Build history of the part. All positions in model axes, mm. A direction names the side the tool comes from. Give positions to 0.01 mm unless a question says otherwise; leave off trailing zeros. Use a Markdown table: item, result. Add a question column.
```python
from build123d import *

# Parameters (mm, degrees)
SKETCH1_R           = 1.5
SKETCH1_R_2         = 1.25
SKETCH1_R_3         = 2.05
BOSS_EXTRUDE1_DEPTH = 2
FILLET7_R           = 8
BOSS_EXTRUDE2_DEPTH = 2
FILLET8_R           = 10
SKETCH4_R           = 1.55
CUT_EXTRUDE1_DEPTH  = 2
SKETCH5_R           = 1.55
CUT_EXTRUDE2_DEPTH  = 2
CUT_EXTRUDE3_DEPTH  = 10
SKETCH7_R           = 1.5
CUT_EXTRUDE4_DEPTH  = 10


with BuildPart() as part:
    # Sketch1 → Boss-Extrude1 (new body)
    with BuildSketch(Plane.XY):
        with BuildLine():
            Line((-86.974134086, 60.104076401), (-60.104076401, 86.974134086))
            Line((-60.104076401, 86.974134086), (60.104076401, 86.974134086))
            Line((60.104076401, 86.974134086), (86.974134086, 60.104076401))
            ThreePointArc((86.974134086, 60.104076401), (73.41582025, 0), (86.974134086, -60.104076401))
            Line((86.974134086, -60.104076401), (60.104076401, -86.974134086))
            Line((60.104076401, -86.974134086), (-60.104076401, -86.974134086))
            Line((-60.104076401, -86.974134086), (-86.974134086, -60.104076401))
            ThreePointArc((-86.974134086, -60.104076401), (-73.41582025, 0), (-86.974134086, 60.104076401))
        make_face()
        with Locations((-15, 57.5)):
            Circle(SKETCH1_R, mode=Mode.SUBTRACT)
        with Locations((-15, 27.5)):
            Circle(SKETCH1_R, mode=Mode.SUBTRACT)
        with Locations((15, 27.5)):
            Circle(SKETCH1_R, mode=Mode.SUBTRACT)
        with Locations((15, 57.5)):
            Circle(SKETCH1_R, mode=Mode.SUBTRACT)
        with Locations((-24, -13.5)):
            Circle(SKETCH1_R_2, mode=Mode.SUBTRACT)
        with Locations((24, -13.5)):
            Circle(SKETCH1_R_2, mode=Mode.SUBTRACT)
        with Locations((24, -46.5)):
            Circle(SKETCH1_R_2, mode=Mode.SUBTRACT)
        with Locations((-24, -46.5)):
            Circle(SKETCH1_R_2, mode=Mode.SUBTRACT)
        with Locations((-76.190755673, 58.159532753)):
            Circle(SKETCH1_R_3, mode=Mode.SUBTRACT)
        with Locations((-58.159532753, 76.190755673)):
            Circle(SKETCH1_R_3, mode=Mode.SUBTRACT)
        with Locations((76.190755673, -58.159532753)):
            Circle(SKETCH1_R_3, mode=Mode.SUBTRACT)
        with Locations((58.159532753, -76.190755673)):
            Circle(SKETCH1_R_3, mode=Mode.SUBTRACT)
        with Locations((-58.159532753, -76.190755673)):
            Circle(SKETCH1_R_3, mode=Mode.SUBTRACT)
        with Locations((-76.190755673, -58.159532753)):
            Circle(SKETCH1_R_3, mode=Mode.SUBTRACT)
        with Locations((58.159532753, 76.190755673)):
            Circle(SKETCH1_R_3, mode=Mode.SUBTRACT)
        with Locations((76.190755673, 58.159532753)):
            Circle(SKETCH1_R_3, mode=Mode.SUBTRACT)
    extrude(amount=BOSS_EXTRUDE1_DEPTH)

    # Fillet7
    fillet7_edges = [part.edges().sort_by_distance(p)[0] for p in [
        (86.974134086, -60.104076401, 1),
        (60.104076401, -86.974134086, 1),
        (-60.104076401, -86.974134086, 1),
        (-86.974134086, -60.104076401, 1),
        (-86.974134086, 60.104076401, 1),
        (-60.104076401, 86.974134086, 1),
        (60.104076401, 86.974134086, 1),
        (86.974134086, 60.104076401, 1),
    ]]
    fillet(fillet7_edges, radius=FILLET7_R)

    # Sketch2 → Boss-Extrude2 (add)
    with BuildSketch(Plane.XY.offset(2)):
        with BuildLine():
            Line((-62.447222151, 84.630988335), (-45.104076401, 101.974134086))
            Line((-45.104076401, 101.974134086), (45.104076401, 101.974134086))
            Line((45.104076401, 101.974134086), (62.447222151, 84.630988335))
            ThreePointArc((62.447222151, 84.630988335), (59.851835361, 86.365170346), (56.790367902, 86.974134086))
            Line((56.790367902, 86.974134086), (-56.790367902, 86.974134086))
            ThreePointArc((-56.790367902, 86.974134086), (-59.851835361, 86.365170346), (-62.447222151, 84.630988335))
        make_face()
    extrude(amount=-BOSS_EXTRUDE2_DEPTH)

    # Fillet8
    fillet8_edges = [part.edges().sort_by_distance(p)[0] for p in [
        (-45.104076401, 101.974134086, 1),
        (45.104076401, 101.974134086, 1),
    ]]
    fillet(fillet8_edges, radius=FILLET8_R)

    # Sketch4 → Cut-Extrude1 (cut)
    with BuildSketch(Plane.XY.offset(2)):
        with Locations((-38.5, -18.5)):
            Circle(SKETCH4_R)
        with Locations((38.5, -18.5)):
            Circle(SKETCH4_R)
        with Locations((38.5, -71.5)):
            Circle(SKETCH4_R)
        with Locations((-38.5, -71.5)):
            Circle(SKETCH4_R)
    extrude(amount=-CUT_EXTRUDE1_DEPTH, mode=Mode.SUBTRACT)

    # Sketch5 → Cut-Extrude2 (cut)
    with BuildSketch(Plane.XY.offset(2)):
        with Locations((-18, 80)):
            Circle(SKETCH5_R)
        with Locations((18, 80)):
            Circle(SKETCH5_R)
        with Locations((18, 10)):
            Circle(SKETCH5_R)
        with Locations((-18, 10)):
            Circle(SKETCH5_R)
    extrude(amount=-CUT_EXTRUDE2_DEPTH, mode=Mode.SUBTRACT)

    # Sketch6 → Cut-Extrude3 (cut)
    with BuildSketch(Plane.XY.offset(2)):
        with BuildLine():
            Line((-40, 45), (-40, 5))
            ThreePointArc((-40, 5), (-49, -4), (-58, 5))
            Line((-58, 5), (-58, 45))
            ThreePointArc((-58, 45), (-49, 54), (-40, 45))
        make_face()
        with BuildLine():
            Line((40, 45), (40, 5))
            ThreePointArc((40, 5), (49, -4), (58, 5))
            Line((58, 5), (58, 45))
            ThreePointArc((58, 45), (49, 54), (40, 45))
        make_face()
        with BuildLine():
            Line((-58.487128717, -25.862080731), (-47.487128717, -46.061090608))
            ThreePointArc((-47.487128717, -46.061090608), (-49.086956522, -51.487005369), (-54.512871283, -49.887177564))
            Line((-54.512871283, -49.887177564), (-65.512871283, -29.688167687))
            ThreePointArc((-65.512871283, -29.688167687), (-63.913043478, -24.262252926), (-58.487128717, -25.862080731))
        make_face()
        with BuildLine():
            Line((58.487128717, -25.862080731), (47.487128717, -46.061090608))
            ThreePointArc((47.487128717, -46.061090608), (49.086956522, -51.487005369), (54.512871283, -49.887177564))
            Line((54.512871283, -49.887177564), (65.512871283, -29.688167687))
            ThreePointArc((65.512871283, -29.688167687), (63.913043478, -24.262252926), (58.487128717, -25.862080731))
        make_face()
    extrude(amount=-CUT_EXTRUDE3_DEPTH, mode=Mode.SUBTRACT)

    # Sketch7 → Cut-Extrude4 (cut)
    with BuildSketch(Plane.XY.offset(2)):
        with Locations((0, 91.974134086)):
            Circle(SKETCH7_R)
        with BuildLine():
            Line((-17.5, 76.974134086), (-7.5, 76.974134086))
            ThreePointArc((-7.5, 76.974134086), (-5.5, 74.974134086), (-7.5, 72.974134086))
            Line((-7.5, 72.974134086), (-17.5, 72.974134086))
            ThreePointArc((-17.5, 72.974134086), (-19.5, 74.974134086), (-17.5, 76.974134086))
        make_face()
        with BuildLine():
            Line((7.5, 76.974134086), (17.5, 76.974134086))
            ThreePointArc((17.5, 76.974134086), (19.5, 74.974134086), (17.5, 72.974134086))
            Line((17.5, 72.974134086), (7.5, 72.974134086))
            ThreePointArc((7.5, 72.974134086), (5.5, 74.974134086), (7.5, 76.974134086))
        make_face()
    extrude(amount=-CUT_EXTRUDE4_DEPTH, mode=Mode.SUBTRACT)


solid = part.part
```
(1) Wall check: probe 1 along Y at (x, z) = (15, 0.7); probe 2 along Y at (x, z) = (-38.5, 1.55); probe 3 along X at (y, z) = (36.5, 0.35). Give the ranges that are in metal, low to high.
(2) Band-saw the part on A-A on z = 0.9. State how many separate pieces and enclosed holes the cut face has, plus the area to 3 significant figures.
(3) Mould opens along X. For faces 3 (the face through (1, 9, 2)), 4 (the face through (73.42, 0.79, 0.99)), 5 (the face through (59.105, -78.009, 0.986)) say: released by +X, released by -X, zero draft, split by the parting line, or undercut.
(4) Tool access for faces 1 (the face through (72.9, -74.18, 0.99)), 2 (the face through (53.064, -35.82, 1.014)): list every direction of +Z, -Z, +X, -X, +Y, -Y with a clear straight run to the whole face (end or side of a thin tool).
Response:
| question | item | result |
|---|---|---|
| 1 | probe 1 | y = -86.97 to 26, 29 to 56, 59 to 72.97, 76.97 to 101.97 |
| 1 | probe 2 | y = -86.97 to -73.05, -69.95 to -20.05, -16.95 to 101.97 |
| 1 | probe 3 | x = -78.26 to -58, -40 to 40, 58 to 78.26 |
| 2 | separate pieces | 1 |
| 2 | enclosed holes | 31 |
| 2 | area | 25,400 mm² |
| 3 | face 3 | zero draft |
| 3 | face 4 | released by +X |
| 3 | face 5 | undercut |
| 4 | face 1 | +Z, -Z, +X, -Y |
| 4 | face 2 | +Z, -Z |
